Design review of the part built by this model. Coordinates are the model's own, in mm. Face numbers are marked on the shaded views. Coordinates: 2 decimals unless noted, no trailing zeros. Loops run counter-clockwise (first coordinate to the right, second up) from the corner with the lowest first, then second, coordinate; pieces in that order, holes last. Notation, with made-up numbers: (-32, 74.5) -> (12, 74.5) arc R23 cw to (12, 94.5) -> close; hole circle Ø8 at (31.5, 84). An arc over 180 degrees is marked (long way). Answer in a Markdown table with one row per item.
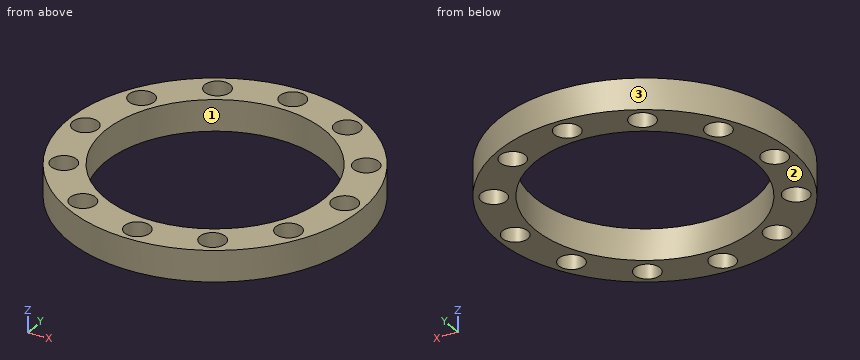
```python
from build123d import *

# Parameters (mm, degrees)
SKETCH1_R           = 330
SKETCH1_R_2         = 247.5
BOSS_EXTRUDE1_DEPTH = 70
SKETCH2_R           = 28.575
CUT_EXTRUDE1_DEPTH  = 131


with BuildPart() as part:
    # Sketch1 → Boss-Extrude1 (new body)
    with BuildSketch(Plane.XY):
        Circle(SKETCH1_R)
        Circle(SKETCH1_R_2, mode=Mode.SUBTRACT)
    extrude(amount=BOSS_EXTRUDE1_DEPTH)

    # Sketch2 → Cut-Extrude1 (cut)
    with BuildSketch(Plane.XY):
        with Locations((0, 290)):
            Circle(SKETCH2_R)
        with Locations((145, 251.147367097)):
            Circle(SKETCH2_R)
        with Locations((251.147367097, 145)):
            Circle(SKETCH2_R)
        with Locations((290, 0)):
            Circle(SKETCH2_R)
        with Locations((251.147367098, -145)):
            Circle(SKETCH2_R)
        with Locations((145, -251.147367097)):
            Circle(SKETCH2_R)
        with Locations((0, -290)):
            Circle(SKETCH2_R)
        with Locations((-145, -251.147367097)):
            Circle(SKETCH2_R)
        with Locations((-251.147367097, -145)):
            Circle(SKETCH2_R)
        with Locations((-290, 0)):
            Circle(SKETCH2_R)
        with Locations((-251.147367097, 145)):
            Circle(SKETCH2_R)
        with Locations((-145, 251.147367097)):
            Circle(SKETCH2_R)
    extrude(amount=CUT_EXTRUDE1_DEPTH, mode=Mode.SUBTRACT)


solid = part.part
```
(1) To check wall thickness, follow probe 1 along X at (y, z) = (-152.5, 50); probe 2 along X at (y, z) = (125, 56); probe 3 along Y at (x, z) = (-155.5, 29.5). State the ranges of each line that lie inside material, in increasing order.
Evaluation:
| item | result |
|---|---|
| probe 1 | x = -292.65 to -278.72, -223.57 to -194.94, 194.94 to 223.57, 278.72 to 292.65 |
| probe 2 | x = -305.41 to -271.56, -230.74 to -213.61, 213.61 to 230.74, 271.56 to 305.41 |
| probe 3 | y = -291.07 to -277.72, -224.57 to -192.55, 192.55 to 224.57, 277.72 to 291.07 |
(2) Take a section at A-A on y = 0. Give the boundary of the cut face in (x, z) (3 decimals).
Evaluation:
| item | result |
|---|---|
| outline | (-330, 0) -> (-318.575, 0) -> (-318.575, 70) -> (-330, 70) -> close; (-261.425, 0) -> (-247.5, 0) -> (-247.5, 70) -> (-261.425, 70) -> close; (247.5, 0) -> (261.425, 0) -> (261.425, 70) -> (247.5, 70) -> close; (318.575, 0) -> (330, 0) -> (330, 70) -> (318.575, 70) -> close |
(3) Take a section at D-D on y = -197. Give the boundary of the cut face in (x, z).
Evaluation:
| item | result |
|---|---|
| outline | (-264.75, 0) -> (-149.82, 0) -> (-149.82, 70) -> (-264.75, 70) -> close; (149.82, 0) -> (264.75, 0) -> (264.75, 70) -> (149.82, 70) -> close |
(4) Take a section at B-B on x = 145. Give the boundary of the cut face in (y, z), and give its area (3 significant figures).
Evaluation:
| item | result |
|---|---|
| outline | (-296.44, 0) -> (-279.72, 0) -> (-279.72, 70) -> (-296.44, 70) -> close; (-222.57, 0) -> (-200.58, 0) -> (-200.58, 70) -> (-222.57, 70) -> close; (200.58, 0) -> (222.57, 0) -> (222.57, 70) -> (200.58, 70) -> close; (279.72, 0) -> (296.44, 0) -> (296.44, 70) -> (279.72, 70) -> close |
| area | 5,420 mm² |
(5) For pin 1 (8 mm diameter, centred on x = -252.5, z = 15, fed in from -Y); pin 2 (8 mm diameter, centred on y = 93.5, z = 46, fed in from -X); pin 3 (8 mm diameter, centred on x = 227.5, z = 18.5, fed in from +Y), all flat-tipped, find the tip position at first contact; note any pin that passes through.
Evaluation:
| item | result |
|---|---|
| pin 1 | stops at y = -217.14 |
| pin 2 | stops at x = -317.63 |
| pin 3 | stops at y = 242.79 |
(6) Take a section at C-C on x = -290. Give the boundary of the cut face in (y, z) (3 decimals), and give its area (3 significant figures).
Evaluation:
| item | result |
|---|---|
| outline | (-157.48, 0) -> (-28.575, 0) -> (-28.575, 70) -> (-157.48, 70) -> close; (28.575, 0) -> (157.48, 0) -> (157.48, 70) -> (28.575, 70) -> close |
| area | 18,000 mm² |
(7) Draft analysis for pull direction X (two halves, no side actions). For the marked faces 1, 2 and 3, state which applies: pulls with the +X half, pulls with the -X half, needs draft (parallel to the pull), parting line crosses it, or undercut.
Evaluation:
| item | result |
|---|---|
| face 1 | undercut |
| face 2 | needs draft |
| face 3 | parting line crosses it |
